Verification items for the finished model (mm, model axes). A direction names the side the tool comes from. Give positions to 0.01 mm unless a question says otherwise; leave off trailing zeros. Loops run counter-clockwise (first coordinate to the right, second up) from the corner with the lowest first, then second, coordinate; pieces in that order, holes last. Notation, with made-up numbers: M 89.5,21 L 100.5,21 A29 cw 100.5,54 Z; hole C -5.5,78 d3. An arc over 180 degrees is marked long. Use a Markdown table: item, result.
from build123d import *

# Parameters (mm, degrees)
SKETCH1_R           = 7.5
BOSS_EXTRUDE1_DEPTH = 14.25
SKETCH2_R           = 7.5
BOSS_EXTRUDE2_DEPTH = 14.25
SKETCH3_R           = 3
CUT_EXTRUDE1_DEPTH  = 32.120732639
SKETCH4_R           = 3
BOSS_EXTRUDE3_DEPTH = 4.25
SKETCH4_2_R         = 3
BOSS_EXTRUDE4_DEPTH = 28.5
SKETCH5_R           = 5
BOSS_EXTRUDE5_DEPTH = 30
SKETCH7_W           = 1
SKETCH7_H           = 2.291482858


with BuildPart() as part:
    # Sketch1 → Boss-Extrude1 (new body)
    with BuildSketch(Plane.XY):
        with Locations(Location((0, -2.5, 0), (0, 0, 180))):
            Circle(SKETCH1_R)
    extrude(amount=BOSS_EXTRUDE1_DEPTH)

    # Sketch2 → Boss-Extrude2 (add)
    with BuildSketch(Plane(origin=(0, 0, 0), x_dir=(-1, 0, 0), z_dir=(0, 0, -1))):
        with Locations(Location((0, 2.5, 0), (0, 0, 199.471220634))):
            Circle(SKETCH2_R)
    extrude(amount=BOSS_EXTRUDE2_DEPTH)

    # Sketch3 → Cut-Extrude1 (cut, through all)
    with BuildSketch(Plane(origin=(0, 0, -14.25), x_dir=(-1, 0, 0), z_dir=(0, 0, -1))):
        Circle(SKETCH3_R)
    extrude(amount=-CUT_EXTRUDE1_DEPTH, mode=Mode.SUBTRACT)



with BuildPart() as body_2:
    # Sketch4 → Boss-Extrude3 (new body)
    with BuildSketch(Plane(origin=(0, 0, -14.25), x_dir=(-1, 0, 0), z_dir=(0, 0, -1))):
        Circle(SKETCH4_R)
    extrude(amount=BOSS_EXTRUDE3_DEPTH)


with BuildPart() as part_1:
    add(part.part)

    add(body_2.part)  # Boss-Extrude4 merges body 2
    # Sketch4<2> → Boss-Extrude4 (add)
    with BuildSketch(Plane(origin=(0, 0, -14.25), x_dir=(-1, 0, 0), z_dir=(0, 0, -1))):
        Circle(SKETCH4_2_R)
    extrude(amount=-BOSS_EXTRUDE4_DEPTH)

    # Sketch5 → Boss-Extrude5 (add)
    with BuildSketch(Plane.XY.offset(14.25)):
        with Locations(Location((0, 0, 0), (0, 0, 89.999372356))):
            Circle(SKETCH5_R)
    extrude(amount=BOSS_EXTRUDE5_DEPTH)

    # Sketch7 → Cut-Revolve1 (revolve, cut)
    with BuildSketch(Plane(origin=(0, 0, 0), x_dir=(0, 0, -1), z_dir=(1, 0, 0))):
        with Locations((-23.75, 5.645741429)):
            Rectangle(SKETCH7_W, SKETCH7_H)
    revolve(axis=Axis((0, 0, 44.25), (0, 0, -1)), mode=Mode.SUBTRACT)


solid = part_1.part
(1) Set-up check for faces 4 (the cylindrical face through (4.88, -1.08, 18.69)), 5 (the cylindrical face through (3, 0, -16)), 6 (the flat face through (-1, 6, 0)), 7 (the flat face through (0, 0, 44.25)): record each of +Z, -Z, +X, -X, +Y, -Y from which the full face is reachable in a straight line by a thin tool's end or side.
Results below:
| item | result |
|---|---|
| face 4 | +Z |
| face 5 | -Z |
| face 6 | +Z, +Y |
| face 7 | +Z, +X, -X, +Y, -Y |
(2) Cross-section at C-C on y = 2.25. Record the cut outline in (x, z), then the cut area to 3 significant figures.
Results below:
| item | result |
|---|---|
| outline | M -7.5,-14.25 L -1.98,-14.25 L -1.98,-18.5 L 1.98,-18.5 L 1.98,-14.25 L 7.5,-14.25 L 7.5,0 L 5.8,0 L 5.8,14.25 L 4.47,14.25 L 4.47,23.25 L 3.9,23.25 L 3.9,24.25 L 4.47,24.25 L 4.47,44.25 L -4.47,44.25 L -4.47,24.25 L -3.9,24.25 L -3.9,23.25 L -4.47,23.25 L -4.47,14.25 L -5.8,14.25 L -5.8,0 L -7.5,0 Z |
| area | 663 mm^2 |
(3) Draft check along Z on faces 1 (the flat face through (0, -6, 14.25)), 2 (the cylindrical face through (4.46, -0.59, 23.74)), 3 (the flat face through (0, 0, -18.5)). Enter one of: +Z half, -Z half, draft (parallel to the pull), parting line (faces both ways), or undercut.
Results below:
| item | result |
|---|---|
| face 1 | +Z half |
| face 2 | undercut |
| face 3 | -Z half |
(4) Cross-section at D-D on z = 35.5. Record the cut outline in (x, y).
Results below:
| item | result |
|---|---|
| outline | C 0,0 d10 |
(5) Cross-section at B-B on z = -6. Record the cut outline in (x, y).
Results below:
| item | result |
|---|---|
| outline | C 0,2.5 d15 |
(6) Cross-section at A-A on y = 7. Record the cut outline in (x, z).
Results below:
| item | result |
|---|---|
| outline | M -6,-14.25 L 6,-14.25 L 6,0 L -6,0 Z |
(7) Gauge pin test, flat ends, axial feed: P1, Ø1, axis at x = -2.5, z = 0, coming from the -Y side; P2, Ø1, axis at x = -0.5, z = 17.5, coming from the -Y side; P3, Ø1, axis at x = 4, y = 5.5, coming from the +Z side. Record the tip position at first contact, or that the pin passes through.
Results below:
| item | result |
|---|---|
| P1 | y = -9.73 |
| P2 | y = -5 |
| P3 | z = 0 |
(8) Material ranges on line 1 (Z direction, x = -6, y = 3); line 2 (Z direction, x = 5.75, y = -1.25); line 3 (Y direction, x = -4, z = 18.5), recorded low to high.
Results below:
| item | result |
|---|---|
| line 1 | -14.25 to 0 |
| line 2 | -14.25 to 14.25 |
| line 3 | -3 to 3 |
